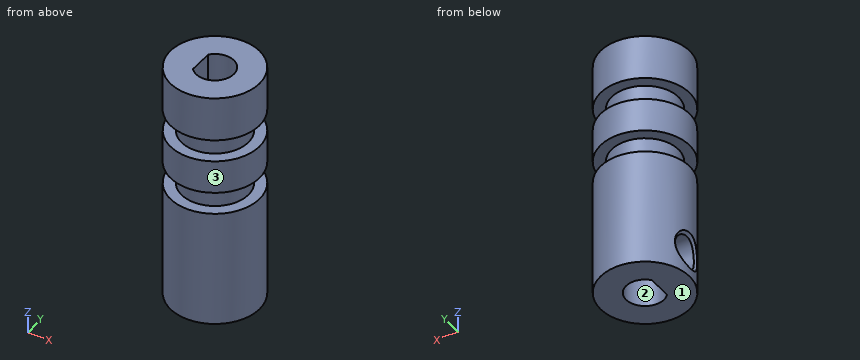
Autodesk Inventor part; units mm, degrees
ref_plane "YZ Plane" through (0, 0, 0) normal (1, 0, 0) x (0, 1, 0)
ref_plane "XZ Plane" through (0, 0, 0) normal (0, 1, 0) x (-1, 0, 0)
ref_plane "XY Plane" through (0, 0, 0) normal (0, 0, 1) x (1, 0, 0)
ref_plane "Work Plane1" through (0, 0, 0.5) normal (0, 0, 1) x (1, 0, 0)
sketch "Sketch1" plane through (0, 0, 0.5) normal (0, 0, 1) x (1, 0, 0)
  arc A0 (13, 1.882) -> (13, 4.118) centre (14, 3) ccw
  arc A1 (13, 1.882) -> (13, 4.118) centre (14, 3) ccw
  line L0 (13, 4.118) -> (13, 1.882)
  circle A2 centre (14, 3) radius 6
  circle A3 centre (14, 3) radius 4
  circle A4 centre (14, 3) radius 1.7
  line L1 (12.7, 1.9046) -> (12.7, 4.0954)
  point P0 (0, 0)
  dimension "d0" = 12
  dimension "d1" = 8
  dimension "d2" = 0.2
  dimension "d3" = 0.3
extrude "Extrusion1" add sketch "Sketch1" along normal blind 21.5 contours A3 | L1 A4 picked at (12.5667, 3)
ref_plane "Work Plane2" through (14, 3, 18) normal (0, 0, 1) x (1, 0, 0)
sketch "Sketch2" plane through (14, 3, 18) normal (0, 0, 1) x (1, 0, 0)
  circle A0 centre (0, 0) radius 4
  arc A1 (-1.3, -1.0954) -> (-1.3, 1.0954) centre (0, 0) ccw
  line L0 (-1.3, -1.0954) -> (-1.3, 1.0954)
  circle A2 centre (0, 0) radius 3
  point P0 (-14, -3)
  dimension "d7" = 6
extrude "Extrusion2" cut sketch "Sketch2" against normal blind 2 contours A0
ref_plane "Work Plane3" through (9.7, 1.9046, 0.5) normal (1, 0, 0) x (0, 0, -1)
sketch "Sketch3" plane through (9.7, 1.9046, 0.5) normal (1, 0, 0) x (0, 0, -1)
  circle A0 centre (-2.5, 1) radius 1.42
  line L0 (-21.5, 0) -> (-21.5, 2.1909)
  point P0 (0.5, -1.9046)
  dimension "d11" = 2.84
  dimension "d12" = 1
  dimension "d15" = 19
extrude "Extrusion3" cut sketch "Sketch3" along normal blind 3
chamfer "Chamfer1" distance 0.25 angle 45 1 edges at (10.0014, 2.8952, 4.42)
ref_plane "Work Plane4" through (14, 3, 13) normal (0, 0, 1) x (1, 0, 0)
sketch "Sketch4" plane through (14, 3, 13) normal (0, 0, 1) x (1, 0, 0)
  circle A0 centre (0, 0) radius 4
  circle A1 centre (0, 0) radius 4
  circle A2 centre (0, 0) radius 3
  point P0 (-14, -3)
extrude "Extrusion4" cut sketch "Sketch4" against normal blind 2
properties part number "rim-v1" material "Tworzywo sztuczne PET"
Read the model definition and answer for the solid it produces. Units are mm, in the model's axes. Face numbers are marked on the shaded views. Give positions to 0.01 mm unless a question says otherwise; leave off trailing zeros. Write each loop counter-clockwise with the first axis right and the second up, starting at its lowest first coordinate (ties: lowest second). Pieces come first, ordered by that corner, then holes. Notation, with made-up numbers: M 17.5,66 L 33.5,66 A31 ccw 33.5,99 Z; hole C -15.75,69 d5. An arc over 180 degrees is marked long. Put each result on its own line as item: value. Start each with the question number.
1. The part is cut by section D-D, the plane x = 15. Give the vertices of the cut face in (y, z).
2. The part is cut by section A-A, the plane x = 14. Give the vertices of the cut face in (y, z), and give its area (3 significant figures).
3. The part is cut by section B-B, the plane y = 6.75. Give the vertices of the cut face in (x, z).
4. Each of these flat-tipped pins is pushed along its axis until it touches: pin 1 Ø2.5 at (y, z) = (2.9, 3) entering from -X; pin 2 Ø0.7 at (y, z) = (2.5, 9.5) entering from +X. Where does it stop, or does it pass through?
5. The part is cut by section C-C, the plane z = 17.25. Give the vertices of the cut face in (x, y).
6. Consider line 1 along Z through (x, y) = (13.75, 6.75); line 2 along X through (y, z) = (3, 10.5); line 3 along Y through (x, z) = (14, 15.25). Determine where each line is inside the solid, lowest interval first.
7. For a pull along Y with two mould halves and no side action, classify the marked faces 1, 2 and 3 as released by +Y, released by -Y, zero draft, split by the parting line, or undercut.
Final values:
1. outline: M -0.87,0.5 L 1.63,0.5 L 1.63,22 L -0.87,22 L -0.87,18 L 0.17,18 L 0.17,16 L -0.87,16 L -0.87,13 L 0.17,13 L 0.17,11 L -0.87,11 Z; M 4.37,0.5 L 6.87,0.5 L 6.87,11 L 5.83,11 L 5.83,13 L 6.87,13 L 6.87,16 L 5.83,16 L 5.83,18 L 6.87,18 L 6.87,22 L 4.37,22 Z
2. outline: M -1,0.5 L 1.3,0.5 L 1.3,22 L -1,22 L -1,18 L 0,18 L 0,16 L -1,16 L -1,13 L 0,13 L 0,11 L -1,11 Z; M 4.7,0.5 L 7,0.5 L 7,11 L 6,11 L 6,13 L 7,13 L 7,16 L 6,16 L 6,18 L 7,18 L 7,22 L 4.7,22 Z
2. area: 90.9 mm²
3. outline: M 12.61,0.5 L 15.39,0.5 L 15.39,11 L 12.61,11 Z; M 12.61,13 L 15.39,13 L 15.39,16 L 12.61,16 Z; M 12.61,18 L 15.39,18 L 15.39,22 L 12.61,22 Z
4. pin 1: stops at x = 12.7
4. pin 2: stops at x = 18
5. outline: C 14,3 d6; hole M 12.7,1.9 A1.7 ccw long 12.7,4.1 Z
6. line 1: z = 0.5 to 11, 13 to 16, 18 to 22
6. line 2: x = 10 to 12.7, 15.7 to 18
6. line 3: y = -1 to 1.3, 4.7 to 7
7. face 1: zero draft
7. face 2: undercut
7. face 3: split by the parting line
